Input: dimensioned drawing with shaded views. Units: mm. Origin: part minimum x, y, z. Give positions to 0.01 mm unless a question says otherwise; leave off trailing zeros. Write each loop counter-clockwise with the first axis right and the second up, starting at its lowest first coordinate (ties: lowest second). Pieces come first, ordered by that corner, then holes.
Q1. Section A-A (x = 500). Return the cut outline in (y, z) (1 decimal).
Q2. Section D-D (x = 178.5). Return the cut outline in (y, z).
Q3. Section C-C (z = 520). Return the cut outline in (x, y).
Q4. Pin query (flat end, axial travel): pin 1 Ø4 at (y, z) = (2.5, 504) entering from -X; pin 2 Ø1.5 at (x, y) = (833.5, 6.5) entering from -Z (1 decimal). Return the tip coordinate at first contact, or that it passes through.
Q5. Line query: line 1 (Z direction, x = 150, y = 6.25) (1 decimal); line 2 (X direction, y = 1, z = 675); line 3 (X direction, y = 8.75, z = 549.5) (1 decimal). Output: solid intervals per line, ascending.
Q6. Section B-B (y = 5.5). State how many separate pieces and enclosed holes the cut face has, plus the area to 3 significant figures.
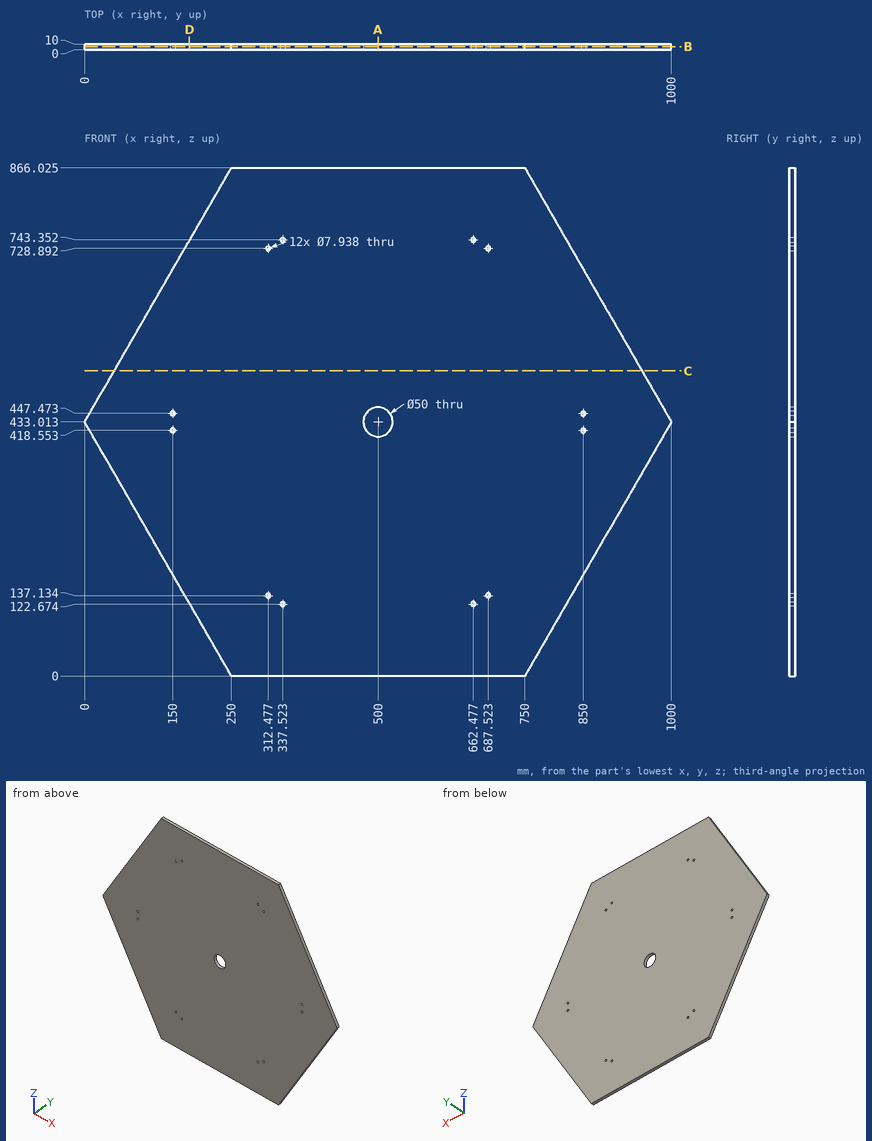
Computed:
1. outline: (0, 0) - (10, 0) - (10, 408) - (0, 408) - close; (0, 458) - (10, 458) - (10, 866) - (0, 866) - close
2. outline: (0, 123.84) - (10, 123.84) - (10, 742.18) - (0, 742.18) - close
3. outline: (50.22, 0) - (949.78, 0) - (949.78, 10) - (50.22, 10) - close
4. pin 1: stops at x = 39.83
4. pin 2: stops at z = 143.3
5. line 1: z = 173.2 to 414.6, 422.5 to 443.5, 451.4 to 692.8
5. line 2: x = 139.71 to 860.29
5. line 3: x = 67.3 to 932.7
6. separate pieces: 1
6. enclosed holes: 13
6. area: 647,000 mm2
